Can you work these out from the model? Positions are in its coordinate system, mm. Face numbers are marked on the shaded views. A direction names the side the tool comes from. Coordinates: 2 decimals unless noted, no trailing zeros. Order: outer loops, then holes, each group sorted by start corner. A loop starts at its lowest first (then second) coordinate and runs counter-clockwise, first axis right, second up. Notation, with made-up numbers: (43.5, 39) - (65.5, 39) arc R23 cw to (65.5, 51) - close; hole circle Ø9 at (44, 62). An arc over 180 degrees is marked (long way). Return JSON: item names as keys, results as strings. Group by question number.
1) Imagine slicing it at B-B (y = 15.5). Write out the boundary of the cut face in (x, z).
2) Imagine slicing it at C-C (x = 22.5). Write out the boundary of the cut face in (y, z), and give its area (3 significant figures).
3) If I drill on line 1 along Y through (x, z) = (22.5, 6.35); line 2 along Z through (x, y) = (7.5, 18.25); line 3 along Z through (x, y) = (14.25, 20), over which ranges is the centre line in solid material (lowest first)?
4) Imagine slicing it at D-D (z = 6). Write out the boundary of the cut face in (x, y), and give its area (3 significant figures).
5) Imagine slicing it at A-A (y = 5). Write out the boundary of the cut face in (x, z).
6) For pin 1 Ø1 at (y, z) = (16, -3) entering from -X; pin 2 Ø3 at (y, z) = (11.5, 7.5) entering from -X; pin 3 Ø4 at (y, z) = (13, -1) entering from +X; pin 4 Ø2 at (x, z) = (9, -1.5) entering from -Y, each with a flat end and sliding along its axis, tell me the tip position at first contact or that it passes through.
7) If we mould it in two halves opening along X, with no side actions, what happens to the marked faces 4, 5, 6 and 7? For each: pulls with the +X half, pulls with the -X half, needs draft (parallel to the pull), parting line crosses it, or undercut.
8) Which directions (+Z, -Z, +X, -X, +Y, -Y) give clear straight access to the entire face, cutting with the end or side of a thin tool? Please do the marked faces 1, 2 and 3.
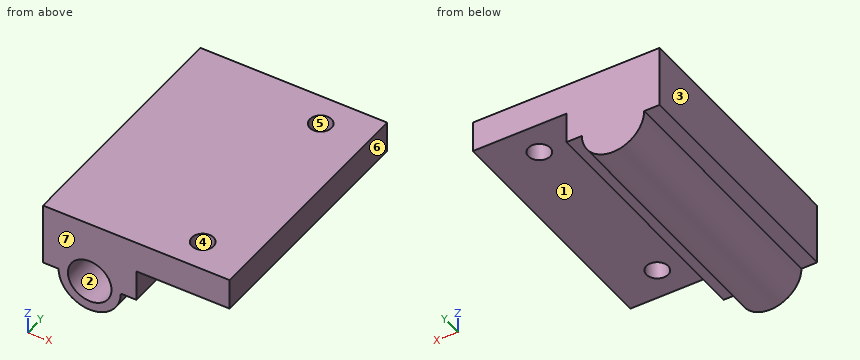
```python
from build123d import *

# Parameters (mm, degrees)
SKETCH1_W           = 30
SKETCH1_H           = 40
BOSS_EXTRUDE1_DEPTH = 10
SKETCH2_W           = 15
SKETCH2_H           = 40
CUT_EXTRUDE1_DEPTH  = 5
SKETCH4_R           = 1.75
CUT_EXTRUDE3_DEPTH  = 30
SKETCH7_R           = 5
BOSS_EXTRUDE2_DEPTH = 40
SKETCH8_R           = 3.5
CUT_EXTRUDE4_DEPTH  = 30


with BuildPart() as part:
    # Sketch1 → Boss-Extrude1 (new body)
    with BuildSketch(Plane.XY):
        with Locations((15, 20)):
            Rectangle(SKETCH1_W, SKETCH1_H)
    extrude(amount=BOSS_EXTRUDE1_DEPTH)

    # Sketch2 → Cut-Extrude1 (cut)
    with BuildSketch(Plane(origin=(0, 0, 0), x_dir=(-1, 0, 0), z_dir=(0, 0, -1))):
        with Locations((-22.5, 20)):
            Rectangle(SKETCH2_W, SKETCH2_H)
    extrude(amount=-CUT_EXTRUDE1_DEPTH, mode=Mode.SUBTRACT)

    # Sketch4 → Cut-Extrude3 (cut)
    with BuildSketch(Plane(origin=(0, 0, 5), x_dir=(-1, 0, 0), z_dir=(0, 0, -1))):
        with Locations((-22.5, 5)):
            Circle(SKETCH4_R)
        with Locations((-22.5, 35)):
            Circle(SKETCH4_R)
    extrude(amount=-CUT_EXTRUDE3_DEPTH, mode=Mode.SUBTRACT)

    # Sketch7 → Boss-Extrude2 (add)
    with BuildSketch(Plane.XZ):
        with Locations((7.5, 0)):
            Circle(SKETCH7_R)
    extrude(amount=-BOSS_EXTRUDE2_DEPTH)

    # Sketch8 → Cut-Extrude4 (cut)
    with BuildSketch(Plane.XZ):
        with Locations((7.5, 0)):
            Circle(SKETCH8_R)
    extrude(amount=-CUT_EXTRUDE4_DEPTH, mode=Mode.SUBTRACT)


solid = part.part
```
Calculated:
{
 "1": {"outline": "(0, 0) - (2.5, 0) arc R5 ccw to (12.5, 0) - (15, 0) - (15, 5) - (30, 5) - (30, 10) - (0, 10) - close; hole circle Ø7 at (7.5, 0)"},
 "2": {"outline": "(0, 5) - (3.25, 5) - (3.25, 10) - (0, 10) - close; (6.75, 5) - (33.25, 5) - (33.25, 10) - (6.75, 10) - close; (36.75, 5) - (40, 5) - (40, 10) - (36.75, 10) - close", "area": "165 mm2"},
 "3": {"line 1": "0 to 3.25, 6.75 to 33.25, 36.75 to 40", "line 2": "-5 to -3.5, 3.5 to 10", "line 3": "0 to 10"},
 "4": {"outline": "(0, 0) - (30, 0) - (30, 40) - (0, 40) - close; hole circle Ø3.5 at (22.5, 5); hole circle Ø3.5 at (22.5, 35)", "area": "1,180 mm2"},
 "5": {"outline": "(0, 0) - (2.5, 0) arc R5 ccw to (12.5, 0) - (15, 0) - (15, 5) - (20.75, 5) - (20.75, 10) - (0, 10) - close; (24.25, 5) - (30, 5) - (30, 10) - (24.25, 10) - close; hole circle Ø7 at (7.5, 0)"},
 "6": {"pin 1": "x = 3.17", "pin 2": "x = 0", "pin 3": "x = 15", "pin 4": "y = 30"},
 "7": {"face 4": "undercut", "face 5": "undercut", "face 6": "pulls with the +X half", "face 7": "needs draft"},
 "8": {"face 1": "-Z, +X, +Y, -Y", "face 2": "-Y", "face 3": "+Z, -Z, -X, +Y, -Y"}
}
